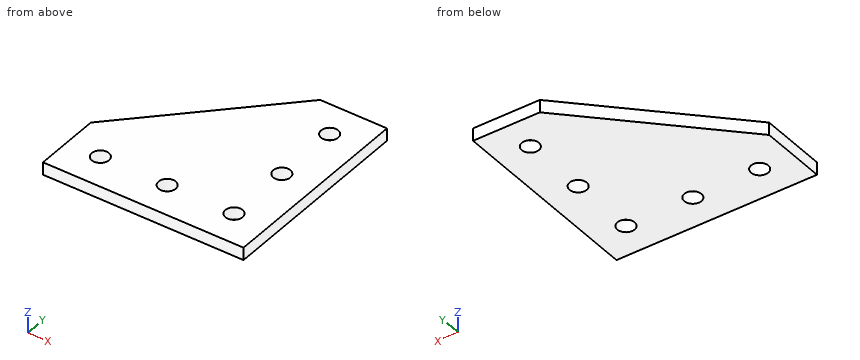
from build123d import *

# Parameters (mm, degrees)
SKETCH1_R           = 3.2639
BOSS_EXTRUDE1_DEPTH = 4.7752


with BuildPart() as part:
    # Sketch1 → Boss-Extrude1 (new body)
    with BuildSketch(Plane.XY):
        Polygon((-63.5, -12.7), (12.7, -12.7), (12.7, 63.5), (-12.7, 63.5), (-63.5, 12.7), align=None)
        with Locations((0, 50.8)):
            Circle(SKETCH1_R, mode=Mode.SUBTRACT)
        with Locations((0, 25.4)):
            Circle(SKETCH1_R, mode=Mode.SUBTRACT)
        Circle(SKETCH1_R, mode=Mode.SUBTRACT)
        with Locations((-25.4, 0)):
            Circle(SKETCH1_R, mode=Mode.SUBTRACT)
        with Locations((-50.8, 0)):
            Circle(SKETCH1_R, mode=Mode.SUBTRACT)
    extrude(amount=BOSS_EXTRUDE1_DEPTH)


solid = part.part
Model file for the job. Use its own axes, mm. Give positions to 0.01 mm unless a question says otherwise; leave off trailing zeros. Loops run counter-clockwise (first coordinate to the right, second up) from the corner with the lowest first, then second, coordinate; pieces in that order, holes last. Notation, with made-up numbers: (-17, 32.25) -> (-12, 32.25) arc R32 cw to (-12, 69.25) -> close; hole circle Ø11 at (52.5, -9.75). An arc over 180 degrees is marked (long way). Use a Markdown table: item, result. Add a question column.
(1) Wall check: line 1 along Y through (x, z) = (0, 3.1); line 2 along X through (y, z) = (-3, 3.05); line 3 along Y through (x, z) = (-2.5, 4.45). Give the ranges that are in metal, low to high.
(2) Slice it at D-D on y = 50.8. List the corners of the cut face in (x, z).
(3) Drop flat-ended pins along their axis: pin 1 Ø5 at (x, y) = (-25.4, 0) entering from -Z; pin 2 Ø2 at (x, z) = (-46, 3.5) entering from +Y. Give the stop position or say it passes through.
(4) Slice it at B-B on x = -25.4. List the corners of the cut face in (y, z), and give its area (3 significant figures).
(5) Slice it at C-C on z = 0.75. List the corners of the cut face in (x, y), and give its area (3 significant figures).
(6) Slice it at A-A on y = 0. List the corners of the cut face in (x, z).
Filled sheet:
| question | item | result |
|---|---|---|
| 1 | line 1 | -12.7 to -3.26, 3.26 to 22.14, 28.66 to 47.54, 54.06 to 63.5 |
| 1 | line 2 | -63.5 to -52.09, -49.51 to -26.69, -24.11 to -1.29, 1.29 to 12.7 |
| 1 | line 3 | -12.7 to -2.1, 2.1 to 23.3, 27.5 to 48.7, 52.9 to 63.5 |
| 2 | outline | (-25.4, 0) -> (-3.26, 0) -> (-3.26, 4.78) -> (-25.4, 4.78) -> close; (3.26, 0) -> (12.7, 0) -> (12.7, 4.78) -> (3.26, 4.78) -> close |
| 3 | pin 1 | through |
| 3 | pin 2 | y = 31.2 |
| 4 | outline | (-12.7, 0) -> (-3.26, 0) -> (-3.26, 4.78) -> (-12.7, 4.78) -> close; (3.26, 0) -> (50.8, 0) -> (50.8, 4.78) -> (3.26, 4.78) -> close |
| 4 | area | 272 mm2 |
| 5 | outline | (-63.5, -12.7) -> (12.7, -12.7) -> (12.7, 63.5) -> (-12.7, 63.5) -> (-63.5, 12.7) -> close; hole circle Ø6.53 at (-50.8, 0); hole circle Ø6.53 at (-25.4, 0); hole circle Ø6.53 at (0, 0); hole circle Ø6.53 at (0, 25.4); hole circle Ø6.53 at (0, 50.8) |
| 5 | area | 4,350 mm2 |
| 6 | outline | (-63.5, 0) -> (-54.06, 0) -> (-54.06, 4.78) -> (-63.5, 4.78) -> close; (-47.54, 0) -> (-28.66, 0) -> (-28.66, 4.78) -> (-47.54, 4.78) -> close; (-22.14, 0) -> (-3.26, 0) -> (-3.26, 4.78) -> (-22.14, 4.78) -> close; (3.26, 0) -> (12.7, 0) -> (12.7, 4.78) -> (3.26, 4.78) -> close |
